Can you work these out from the model? Positions are in its coordinate system, mm. Face numbers are marked on the shaded views. Round coordinates to 2 decimals unless told otherwise and drop trailing zeros. Order: outer loops, then holes, each group sorted by start corner. A loop starts at its lowest first (then second) coordinate and runs counter-clockwise, first axis right, second up.
Q1. If we section it at A-A (y = 118.5): Please give me the cut outline in (x, z), plus the area to 3 significant figures.
Q2. Will these pins go through, and if not, where does the flat tip stop? P1, Ø3, axis at x = 8.5, z = 6.5, coming from the -Y side; P2, Ø4, axis at y = 223, z = 2, coming from the -X side; P3, Ø1.5, axis at x = -5, z = 1.5, coming from the -Y side; P4, Ø12.5, axis at x = 0, y = 240, coming from the -Z side.
Q3. If we section it at B-B (z = 6.25): Count the separate pieces of the cut face and the enclosed holes in it, plus the area to 3 significant figures.
Q4. If we section it at C-C (y = 17.5): Please give me the cut outline in (x, z).
Q5. If I drill on line 1 (Y direction, x = -6, z = 1.5); line 2 (X direction, y = 85, z = 2); line 3 (Y direction, x = 20.5, z = 10.75), over which ranges is the centre line in solid material (lowest first)?
Q6. We'd pull the mould along X, two halves only. Please class the marked faces 1, 2 and 3: pulls with the +X half, pulls with the -X half, needs draft (parallel to the pull), parting line crosses it, or undercut.
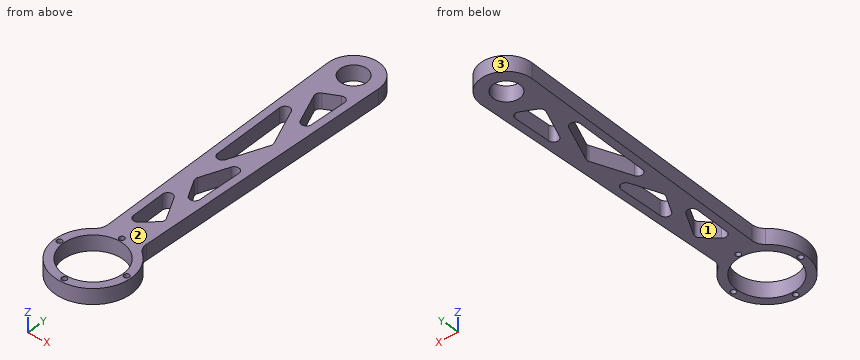
from build123d import *

# Parameters (mm, degrees)
EXTRUDE_1_DEPTH     = 12
SKETCH_2_R          = 10.5
SKETCH_2_R_2        = 23.5
CUT_EXTRUDE_1_DEPTH = 39
FILLET_1_R          = 10
SKETCH_3_R          = 2.1
CUT_EXTRUDE_2_DEPTH = 68
CUT_EXTRUDE_3_DEPTH = 263
FILLET_3_R          = 4


with BuildPart() as part:
    # 草图1 → 凸台-拉伸1 (new body)
    with BuildSketch(Plane.XY):
        with BuildLine():
            Line((-15, 25.980762114), (-19.994532285, 239.532369068))
            ThreePointArc((-19.994532285, 239.532369068), (0, 260), (19.994532285, 239.532369068))
            Line((19.994532285, 239.532369068), (15, 25.980762114))
            ThreePointArc((15, 25.980762114), (0, -30), (-15, 25.980762114))
        make_face()
    extrude(amount=EXTRUDE_1_DEPTH)

    # 草图2 → 切除-拉伸1 (cut)
    with BuildSketch(Plane.XY.offset(12)):
        with Locations((0, 240)):
            Circle(SKETCH_2_R)
        Circle(SKETCH_2_R_2)
    extrude(amount=-CUT_EXTRUDE_1_DEPTH, mode=Mode.SUBTRACT)

    # 圆角1
    fillet_1_edges = [part.edges().sort_by_distance(p)[0] for p in [
        (15, 25.980762114, 6),
        (-15, 25.980762114, 6),
    ]]
    fillet(fillet_1_edges, radius=FILLET_1_R)

    # 草图3 → 切除-拉伸2 (cut)
    with BuildSketch(Plane.XY.offset(12)):
        with Locations((0, 26.5)):
            Circle(SKETCH_3_R)
        with Locations((26.5, 0)):
            Circle(SKETCH_3_R)
        with Locations((0, -26.5)):
            Circle(SKETCH_3_R)
        with Locations((-26.5, 0)):
            Circle(SKETCH_3_R)
    extrude(amount=-CUT_EXTRUDE_2_DEPTH, mode=Mode.SUBTRACT)

    # 草图6 → 切除-拉伸3 (cut, through all)
    with BuildSketch(Plane(origin=(0, 0, 0), x_dir=(-1, 0, 0), z_dir=(0, 0, -1))):
        Polygon((-13.597448285, 222.62437169), (6.396098914, 212.643766677), (-12.305308581, 167.376253439), align=None)
        Polygon((13.262733731, 208.312955361), (-8.237709541, 156.270262815), (10.920628657, 108.171385833), align=None)
        Polygon((-11.745923389, 143.458577117), (5.525281493, 100.097532419), (-10.051201509, 70.997221333), align=None)
        Polygon((-8.948192405, 56.105719255), (10.555093379, 92.542165366), (9.310631693, 39.332619917), align=None)
    extrude(amount=-CUT_EXTRUDE_3_DEPTH, mode=Mode.SUBTRACT)

    # 圆角3
    fillet_3_edges = [part.edges().sort_by_distance(p)[0] for p in [
        (10.051201509, 70.997221333, 6),
        (11.745923389, 143.458577117, 6),
        (-5.525281493, 100.097532419, 6),
        (-13.262733731, 208.312955361, 6),
        (-10.920628657, 108.171385833, 6),
        (8.237709541, 156.270262815, 6),
        (-9.310631693, 39.332619917, 6),
        (8.948192405, 56.105719255, 6),
        (-10.555093379, 92.542165366, 6),
        (12.305308581, 167.376253439, 6),
        (13.597448285, 222.62437169, 6),
        (-6.396098914, 212.643766677, 6),
    ]]
    fillet(fillet_3_edges, radius=FILLET_3_R)


solid = part.part
Solution:
1. outline: (-17.16, 0) - (1.8, 0) - (1.8, 12) - (-17.16, 12) - close; (11.16, 0) - (17.16, 0) - (17.16, 12) - (11.16, 12) - close
1. area: 300 mm2
2. P1: stops at y = -29.17
2. P2: stops at x = -19.65
2. P3: stops at y = -29.7
2. P4: passes through
3. separate pieces: 1
3. enclosed holes: 10
3. area: 6,450 mm2
4. outline: (-24.37, 0) - (-15.68, 0) - (-15.68, 12) - (-24.37, 12) - close; (15.68, 0) - (24.37, 0) - (24.37, 12) - (15.68, 12) - close
5. line 1: y = -29.39 to -22.72, 22.72 to 44.28, 79.86 to 124.12, 189.84 to 231.38, 248.62 to 259.08
5. line 2: x = -16.38 to 2.56, 10.2 to 16.38
5. line 3: y = -21.9 to -11.49, 11.49 to 21.9
6. face 1: undercut
6. face 2: needs draft
6. face 3: parting line crosses it
